Input: part model. Units: mm. Frame: model coordinates. A direction names the side the tool comes from. Give positions to 0.01 mm unless a question says otherwise; leave off trailing zeros. Order: outer loops, then holes, each group sorted by start corner. A loop starts at its lowest first (then second) coordinate and runs counter-clockwise, first axis right, second up. Notation, with made-up numbers: M 2.25,60.5 L 7.25,60.5 A21 cw 7.25,97.5 Z; hole C 15.5,89 d9. An arc over 180 degrees is marked long. Use a Markdown table: item, result.
from build123d import *

# Parameters (mm, degrees)
F0_R     = 63.5
F1_DEPTH = 457.2
F1_TAPER = -3
F2_R     = 57.15
F2_R_2   = 50.8
F3_DEPTH = 5.08
F4_R     = 78.74
F4_R_2   = 76.2
F5_DEPTH = 25.4


with BuildPart() as f1:
    # F0 (on Top) → F1 (new body)
    with BuildSketch(Plane.XY):
        Circle(F0_R)
    extrude(amount=F1_DEPTH, taper=F1_TAPER)

    # F2 (on face) → F3 (join)
    with BuildSketch(Plane(origin=(0, 0, 0), x_dir=(1, 0, 0), z_dir=(0, 0, -1))):
        Circle(F2_R)
        Circle(F2_R_2, mode=Mode.SUBTRACT)
    extrude(amount=F3_DEPTH)

    # F4 (on face) → F5 (join)
    with BuildSketch(Plane.XY.offset(457.2)):
        Circle(F4_R)
        Circle(F4_R_2, mode=Mode.SUBTRACT)
    extrude(amount=F5_DEPTH)


solid = f1.part
1) Cut plane A-A on x = 0. Return loops of the section in (y, z), and give its area (3 significant figures).
Response values:
| item | result |
|---|---|
| outline | M -87.46,457.2 L -63.5,0 L -57.15,0 L -57.15,-5.08 L -50.8,-5.08 L -50.8,0 L 50.8,0 L 50.8,-5.08 L 57.15,-5.08 L 57.15,0 L 63.5,0 L 87.46,457.2 L 78.74,457.2 L 78.74,482.6 L 76.2,482.6 L 76.2,457.2 L -76.2,457.2 L -76.2,482.6 L -78.74,482.6 L -78.74,457.2 Z |
| area | 69,200 mm² |
2) Mould query, pull axis X, two halves, no side actions, for faces 4 (the face through (-1, 1, 0)), 5 (the face through (-16.4, -73.85, 231.8)), 6 (the face through (-41, 65, 482.6)). Classes: released by +X, released by -X, zero draft, split by the parting line, or undercut.
Response values:
| item | result |
|---|---|
| face 4 | undercut |
| face 5 | split by the parting line |
| face 6 | zero draft |
3) First-contact query: pin 1 Ø2 at (y, z) = (-20.5, 304) entering from -X; pin 2 Ø8 at (y, z) = (4.5, 94.5) entering from -X; pin 3 Ø8 at (x, z) = (69, 235) entering from +Y. Flat tips, straight axial feed; report the tip coordinate or a pass-through.
Response values:
| item | result |
|---|---|
| pin 1 | stops at x = -77.01 |
| pin 2 | stops at x = -68.59 |
| pin 3 | stops at y = 39.04 |
4) Cut plane B-B on z = 449. Return loops of the section in (x, y).
Response values:
| item | result |
|---|---|
| outline | C 0,0 d174.06 |
5) Cut plane C-C on z = 250. Return loops of the section in (x, y).
Response values:
| item | result |
|---|---|
| outline | C 0,0 d153.2 |
6) Reachability of faces 1 (the face through (-38, 34, -5.08)), 2 (the face through (-1, 1, 457.2)), 3 (the face through (-11.012, 49.592, -2.504)) from +Z, -Z, +X, -X, +Y, -Y: full face, straight path, thin tool, end or side. Return the list, or none.
Response values:
| item | result |
|---|---|
| face 1 | -Z, +X, -X, +Y, -Y |
| face 2 | +Z |
| face 3 | -Z |
7) Material intervals for line 1 (Y direction, x = 0, z = 468.25); line 2 (Y direction, x = 0, z = -1); line 3 (Z direction, x = 32, y = 2.5), sorted ascending. Write a range as from..to.
Response values:
| item | result |
|---|---|
| line 1 | y = -78.74..-76.2, 76.2..78.74 |
| line 2 | y = -57.15..-50.8, 50.8..57.15 |
| line 3 | z = 0..457.2 |
